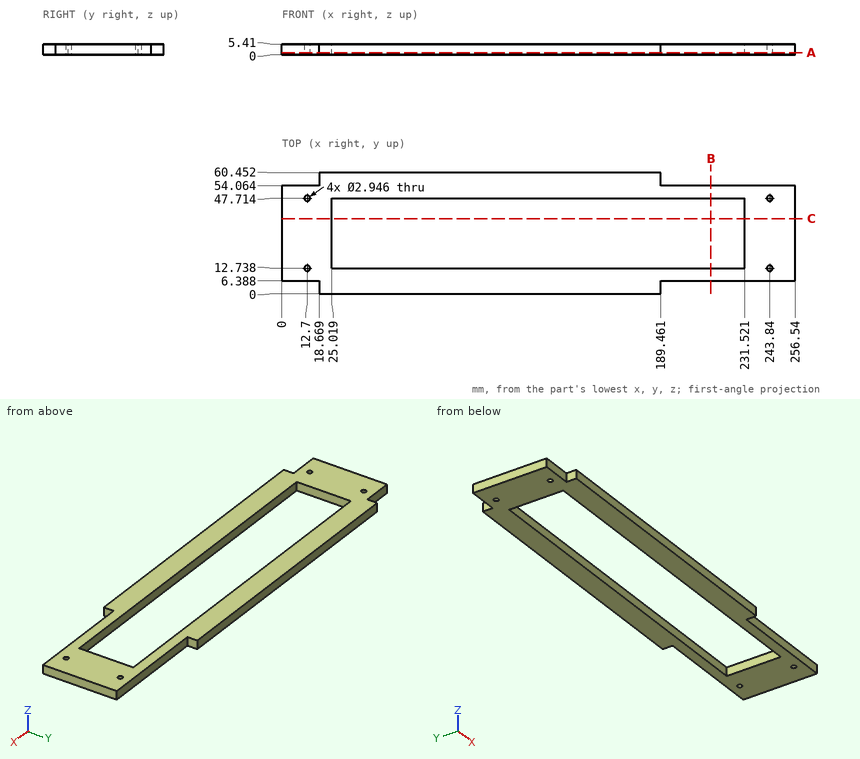
Design review of the part shown in the three views and the two pictorial views. Dimensions are in mm from the part's minimum x, y and z. Coordinates: 2 decimals unless noted, no trailing zeros. Write each loop counter-clockwise with the first axis right and the second up, starting at its lowest first coordinate (ties: lowest second). Pieces come first, ordered by that corner, then holes. Notation, with made-up numbers: (1.25, 51) - (28.25, 51) arc R18 ccw to (28.25, 73) - close; hole circle Ø1 at (41, 85). An arc over 180 degrees is marked (long way). Write item = value, one per line.
(1) For P1, Ø2.5, axis at x = 224.5, z = 3, coming from the +Y side; P2, Ø2.5, axis at x = 12.7, y = 12.74, coming from the -Z side; P3, Ø2.5, axis at x = 11.5, z = 2.5, coming from the -Y side; P4, Ø2.5, axis at y = 56, z = 1.5, coming from the -X side, all flat-tipped, find the tip position at first contact; note any pin that passes through.
Result sheet:
P1 = 54.06
P2 = through
P3 = 6.39
P4 = 18.67
(2) For line 1 (Y direction, x = 12.7, z = 3.5) (1 decimal); line 2 (Y direction, x = 130.5, z = 3.3); line 3 (X direction, y = 40.5, z = 4.7), list the stretches that pass through material, from the lowest coordinate up. Write a range as [from, to].
Result sheet:
line_1 = [6.4, 11.3], [14.2, 46.2], [49.2, 54.1]
line_2 = [0, 12.74], [47.71, 60.45]
line_3 = [0, 25.02], [231.52, 256.54]
(3) Consider section A-A, the plane z = 1.1. Give the boundary of the cut face in (x, y).
Result sheet:
outline = (0, 6.39) - (18.67, 6.39) - (18.67, 0) - (189.46, 0) - (189.46, 6.39) - (256.54, 6.39) - (256.54, 54.06) - (189.46, 54.06) - (189.46, 60.45) - (18.67, 60.45) - (18.67, 54.06) - (0, 54.06) - close; hole circle Ø2.95 at (12.7, 12.74); hole circle Ø2.95 at (12.7, 47.71); hole (25.02, 12.74) - (231.52, 12.74) - (231.52, 47.71) - (25.02, 47.71) - close; hole circle Ø2.95 at (243.84, 12.74); hole circle Ø2.95 at (243.84, 47.71)
(4) Consider section C-C, the plane y = 37.5. Give the boundary of the cut face in (x, z), then the cut area to 3 significant figures.
Result sheet:
outline = (0, 0) - (25.02, 0) - (25.02, 5.41) - (0, 5.41) - close; (231.52, 0) - (256.54, 0) - (256.54, 5.41) - (231.52, 5.41) - close
area = 271 mm^2
(5) Consider section B-B, the plane x = 214.5. Give the boundary of the cut face in (y, z).
Result sheet:
outline = (6.39, 0) - (12.74, 0) - (12.74, 5.41) - (6.39, 5.41) - close; (47.71, 0) - (54.06, 0) - (54.06, 5.41) - (47.71, 5.41) - close
